The model under review builds one solid part; all positions refer to its coordinate system, in mm. Face numbers are marked on the shaded views. Give positions to 0.01 mm unless a question says otherwise; leave off trailing zeros. Write each loop counter-clockwise with the first axis right and the second up, starting at its lowest first coordinate (ties: lowest second). Pieces come first, ordered by that corner, then holes. Notation, with made-up numbers: (38, 64.25) - (49, 64.25) arc R16 ccw to (49, 69.25) - close; hole circle Ø4 at (-39, -17.5). An arc over 180 degrees is marked (long way). Write item = value, one per line.
```python
from build123d import *

# Parameters (mm, degrees)
BOSS_EXTRUDE1_DEPTH         = 16.51
BOSS_EXTRUDE2_DEPTH         = 1.778
F_1_4_0_25_DIAMETER_HOLE1_D = 6.35
SKETCH6_W                   = 53.975
SKETCH6_H                   = 44.45
CUT_EXTRUDE1_DEPTH          = 14.2875
F_0_257_DIAMETER_HOLE1_D    = 6.5278


with BuildPart() as part:
    # Sketch1 → Boss-Extrude1 (new, symmetric)
    with BuildSketch(Plane.XY):
        with BuildLine():
            Line((25.4, 19.05), (-25.4, 19.05))
            Line((-25.4, 19.05), (-5.720931214, -21.805620809))
            ThreePointArc((-5.720931214, -21.805620809), (0, -25.4), (5.720931214, -21.805620809))
            Line((5.720931214, -21.805620809), (25.4, 19.05))
        make_face()
    extrude(amount=BOSS_EXTRUDE1_DEPTH, both=True)

    # Sketch2 → Boss-Extrude2 (add)
    with BuildSketch(Plane(origin=(0, 19.05, 0), x_dir=(1, 0, 0), z_dir=(0, 1, 0))):
        Polygon((-34.036, -20.574), (-34.036, 20.574), (-23.368, 20.574), (-23.368, 16.51), (23.368, 16.51), (23.368, 20.574), (34.036, 20.574), (34.036, -20.574), (23.368, -20.574), (23.368, -16.51), (-23.368, -16.51), (-23.368, -20.574), align=None)
    extrude(amount=-BOSS_EXTRUDE2_DEPTH)

    # 1/4 (0.25) Diameter Hole1 (through all)
    with Locations(Plane(origin=(0, 19.05, 0), x_dir=(1, 0, 0), z_dir=(0, 1, 0))):
        with Locations((-26.797, 14.603831543), (-26.797, -14.603831543), (26.797, -14.603831543), (26.797, 14.603831543)):
            Hole(F_1_4_0_25_DIAMETER_HOLE1_D / 2)

    # Sketch6 → Cut-Extrude1 (cut, symmetric)
    with BuildSketch(Plane.XY):
        with Locations((0, -4.953)):
            Rectangle(SKETCH6_W, SKETCH6_H)
    extrude(amount=CUT_EXTRUDE1_DEPTH, both=True, mode=Mode.SUBTRACT)

    # F (0.257) Diameter Hole1 (through all)
    with Locations(Plane.XY.offset(16.51)):
        with Locations((0, -19.05)):
            Hole(F_0_257_DIAMETER_HOLE1_D / 2)


solid = part.part
```
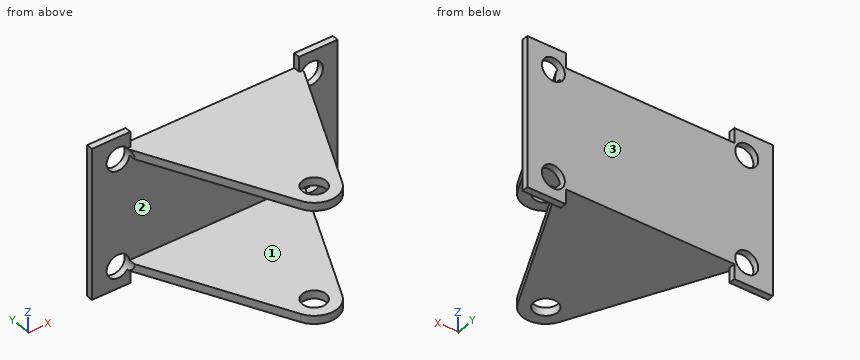
1. Take a section at A-A on x = 0. Give the boundary of the cut face in (y, z).
Findings below:
outline = (-25.4, -16.51) - (-22.31, -16.51) - (-22.31, -14.29) - (-25.4, -14.29) - close; (-25.4, 14.29) - (-22.31, 14.29) - (-22.31, 16.51) - (-25.4, 16.51) - close; (-15.79, -16.51) - (19.05, -16.51) - (19.05, 16.51) - (-15.79, 16.51) - (-15.79, 14.29) - (17.27, 14.29) - (17.27, -14.29) - (-15.79, -14.29) - close
2. Take a section at C-C on z = -13. Give the boundary of the cut face in (x, y), and give its area (3 significant figures).
Findings below:
outline = (-34.04, 17.27) - (-29.54, 17.27) - (-29.54, 19.05) - (-34.04, 19.05) - close; (-24.06, 17.27) - (24.06, 17.27) - (24.06, 19.05) - (-24.06, 19.05) - close; (29.54, 17.27) - (34.04, 17.27) - (34.04, 19.05) - (29.54, 19.05) - close
area = 102 mm²
3. Insertion check: P1, Ø7.5, axis at x = 26.8, z = -14.6, coming from the +Y side; P2, Ø12.5, axis at x = -3.5, z = -5.5, coming from the -Y side; P3, Ø21.5, axis at x = 3, y = -12, coming from the +Z side; P4, Ø3, axis at x = 5.5, y = 11.5, coming from the -Z side. Each pin has a flat end and moves straight along its axis. Give the tip position at first contact, or say it passes through.
Findings below:
P1 = 19.05
P2 = 17.27
P3 = 16.51
P4 = -16.51
4. Take a section at B-B on y = 8.5. Give the boundary of the cut face in (x, z), and give its area (3 significant figures).
Findings below:
outline = (-20.32, -16.51) - (20.32, -16.51) - (20.32, -14.29) - (-20.32, -14.29) - close; (-20.32, 14.29) - (20.32, 14.29) - (20.32, 16.51) - (-20.32, 16.51) - close
area = 181 mm²
5. Draft analysis for pull direction Z (two halves, no side actions). For the marked faces 1, 2 and 3, state which applies: +Z half, -Z half, draft (parallel to the pull), parting line (faces both ways), or undercut.
Findings below:
face_1 = undercut
face_2 = undercut
face_3 = draft
6. Take a section at D-D on y = -17. Give the boundary of the cut face in (x, z).
Findings below:
outline = (-8.04, -16.51) - (-2.54, -16.51) - (-2.54, -14.29) - (-8.04, -14.29) - close; (-8.04, 14.29) - (-2.54, 14.29) - (-2.54, 16.51) - (-8.04, 16.51) - close; (2.54, -16.51) - (8.04, -16.51) - (8.04, -14.29) - (2.54, -14.29) - close; (2.54, 14.29) - (8.04, 14.29) - (8.04, 16.51) - (2.54, 16.51) - close
7. For line 1 (Z direction, x = 6, y = -21); line 2 (Y direction, x = 0, z = 14.9); line 3 (Y direction, x = 30.5, z = 19.5), list the stretches that pass through material, from the lowest coordinate up. Write a range as from..to.
Findings below:
line_1 = -16.51..-14.29, 14.29..16.51
line_2 = -25.4..-22.31, -15.79..19.05
line_3 = 17.27..19.05
